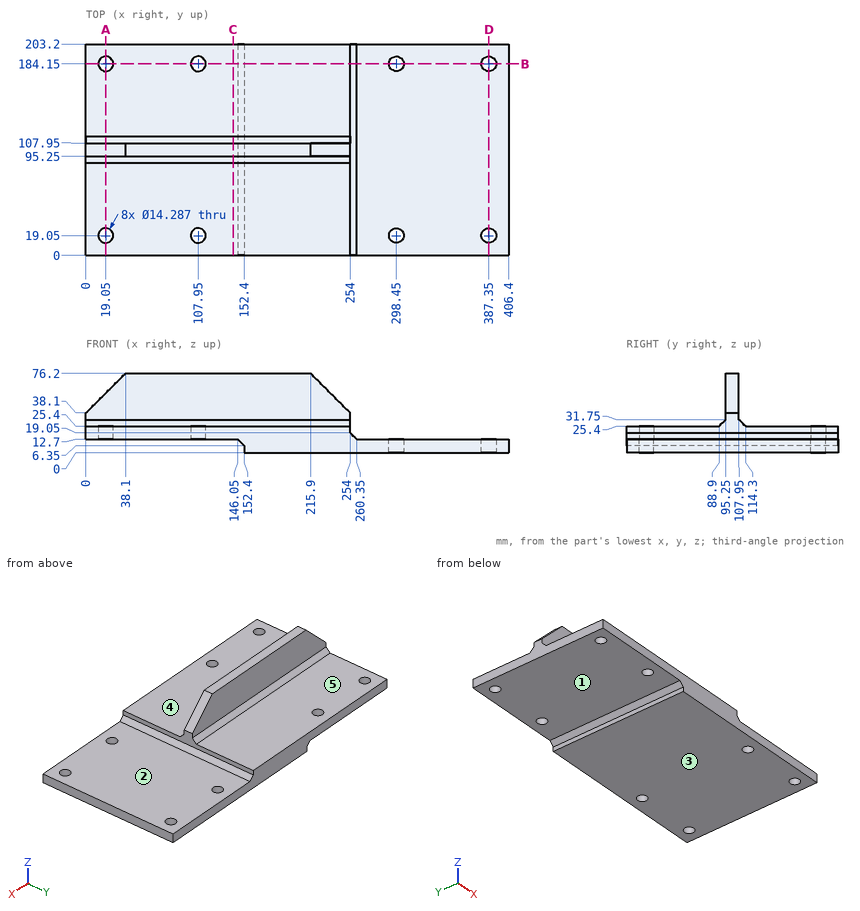
Input: dimensioned drawing with shaded views. Units: mm. Origin: part minimum x, y, z. A direction names the side the tool comes from. Coordinates: 2 decimals unless noted, no trailing zeros. Loops run counter-clockwise (first coordinate to the right, second up) from the corner with the lowest first, then second, coordinate; pieces in that order, holes last. Notation, with made-up numbers: (13, -12.75) -> (43, -12.75) arc R22 ccw to (43, 11.25) -> close; hole circle Ø8 at (45, 75.25). An arc over 180 degrees is marked (long way). One line per item, written item: value. Start each with the question number.
Q1. Section query C-C, the plane x = 141.5. Return the cut outline in (y, z).
Q2. Section query D-D, the plane x = 387.35. Return the cut outline in (y, z), and give its area (3 significant figures).
Q3. Contact query for flat-ended pins moving along their axis: P1, Ø6, axis at x = 174.5, y = 113, coming from the +Z side; P2, Ø13, axis at x = 298.45, y = 184.15, coming from the +Z side; P3, Ø2, axis at y = 68, z = 14, coming from the -X side; P4, Ø22, axis at x = 97, z = 58.5, coming from the -Y side. Output: stop coordinate, or through.
Q4. Line query: line 1 along Y through (x, z) = (387.35, 4.5); line 2 along X through (y, z) = (19, 4); line 3 along Y through (x, z) = (122, 38). Output: solid intervals per line, ascending.
Q5. Section query B-B, the plane y = 184.15. Return the cut outline in (x, z).
Q6. Section query A-A, the plane x = 19.05. Return the cut outline in (y, z), and give its area (3 significant figures).
Q7. Set-up query: the marked faces 1, 2, 3, 4 and 5. Return all of +Z, -Z, +X, -X, +Y, -Y with unobstructed straight access to the full face (end or side cutting, diameter ignored); none if empty.
Results:
1. outline: (0, 12.7) -> (203.2, 12.7) -> (203.2, 25.4) -> (114.3, 25.4) -> (107.95, 31.75) -> (107.95, 76.2) -> (95.25, 76.2) -> (95.25, 31.75) -> (88.9, 25.4) -> (0, 25.4) -> close
2. outline: (0, 0) -> (11.91, 0) -> (11.91, 12.7) -> (0, 12.7) -> close; (26.19, 0) -> (177.01, 0) -> (177.01, 12.7) -> (26.19, 12.7) -> close; (191.29, 0) -> (203.2, 0) -> (203.2, 12.7) -> (191.29, 12.7) -> close
2. area: 2,220 mm^2
3. P1: z = 29.7
3. P2: through
3. P3: x = 0
3. P4: y = 95.25
4. line 1: 0 to 11.91, 26.19 to 177.01, 191.29 to 203.2
4. line 2: 152.4 to 291.31, 305.59 to 380.21, 394.49 to 406.4
4. line 3: 95.25 to 107.95
5. outline: (0, 12.7) -> (11.91, 12.7) -> (11.91, 25.4) -> (0, 25.4) -> close; (26.19, 12.7) -> (100.81, 12.7) -> (100.81, 25.4) -> (26.19, 25.4) -> close; (115.09, 12.7) -> (146.05, 12.7) -> (152.4, 6.35) -> (152.4, 0) -> (291.31, 0) -> (291.31, 12.7) -> (260.35, 12.7) -> (254, 19.05) -> (254, 25.4) -> (115.09, 25.4) -> close; (305.59, 0) -> (380.21, 0) -> (380.21, 12.7) -> (305.59, 12.7) -> close; (394.49, 0) -> (406.4, 0) -> (406.4, 12.7) -> (394.49, 12.7) -> close
6. outline: (0, 12.7) -> (11.91, 12.7) -> (11.91, 25.4) -> (0, 25.4) -> close; (26.19, 12.7) -> (177.01, 12.7) -> (177.01, 25.4) -> (114.3, 25.4) -> (107.95, 31.75) -> (107.95, 57.15) -> (95.25, 57.15) -> (95.25, 31.75) -> (88.9, 25.4) -> (26.19, 25.4) -> close; (191.29, 12.7) -> (203.2, 12.7) -> (203.2, 25.4) -> (191.29, 25.4) -> close
6. area: 2,660 mm^2
7. face 1: -Z, -X, +Y, -Y
7. face 2: +Z, +X, +Y, -Y
7. face 3: -Z, +X, -X, +Y, -Y
7. face 4: +Z, +X, -X, -Y
7. face 5: +Z, +X, -X, +Y
